from build123d import *

# Parameters (mm, degrees)
F1_DEPTH = 1
F3_W     = 140
F3_H     = 1
F4_DEPTH = 2
F6_DEPTH = 1


with BuildPart() as f1:
    # F0 (on Top) → F1 (new body)
    with BuildSketch(Plane.XY):
        Polygon((-20, 0), (0, 0), (0, 180), (-70, 180), (-70, 110), align=None)
        with BuildLine():
            ThreePointArc((-58.549692, 120), (-62.817459, 118.232233), (-61.049692, 122.5))
            ThreePointArc((-61.049692, 122.5), (-59.281925, 121.767767), (-58.549692, 120))
        make_face(mode=Mode.SUBTRACT)
        with BuildLine():
            ThreePointArc((-32.549692, 120), (-35.049692, 117.5), (-37.549692, 120))
            ThreePointArc((-37.549692, 120), (-36.817459, 121.767767), (-35.049692, 122.5))
            ThreePointArc((-35.049692, 122.5), (-33.281925, 121.767767), (-32.549692, 120))
        make_face(mode=Mode.SUBTRACT)
        with BuildLine():
            ThreePointArc((-61.049692, 170.5), (-62.817459, 174.767767), (-58.549692, 173))
            ThreePointArc((-58.549692, 173), (-59.281925, 171.232233), (-61.049692, 170.5))
        make_face(mode=Mode.SUBTRACT)
        with BuildLine():
            ThreePointArc((-32.549692, 173), (-33.281925, 171.232233), (-35.049692, 170.5))
            ThreePointArc((-35.049692, 170.5), (-36.817459, 174.767767), (-32.549692, 173))
        make_face(mode=Mode.SUBTRACT)
    extrude(amount=F1_DEPTH)

    # F2: F1 across face


with BuildPart() as f1_1:
    add(f1.part)
    add(f1.part.mirror(Plane(origin=(0, 90, 0.5), x_dir=(0, 1, 0), z_dir=(1, 0, 0))))

    # F3 (on face) → F4 (join)
    with BuildSketch(Plane.XY.offset(1)):
        with Locations((0, 179.5)):
            Rectangle(F3_W, F3_H)
    extrude(amount=F4_DEPTH)

    # F5 (on face) → F6 (join)
    with BuildSketch(Plane.XY.offset(1)):
        Polygon((-69, 110.216609), (-69, 179), (-70, 179), (-70, 110), (-20, 0), (-16.780434, 0), (16.780434, 0), (20, 0), (70, 110), (70, 179), (69, 179), (69, 110.216609), (19.356087, 1), (-19.356087, 1), align=None)
    extrude(amount=F6_DEPTH)


solid = f1_1.part
Read the model definition and answer for the solid it produces. Units are mm, in the model's axes. A direction names the side the tool comes from. Coordinates: 2 decimals unless noted, no trailing zeros. Order: outer loops, then holes, each group sorted by start corner. A loop starts at its lowest first (then second) coordinate and runs counter-clockwise, first axis right, second up. Notation, with made-up numbers: M 18,-23 L 59,-23 A17 ccw 59,-14 Z; hole C 57,6.5 d5. An arc over 180 degrees is marked long. Put each result on its own line as item: value. Start each with the question number.
Item 1: Section B-B, the plane x = 50 is taken. Determine the outline of the cut face in (y, z).
Item 2: Section A-A, the plane y = 88 is taken. Determine the outline of the cut face in (x, z), plus the area to 3 significant figures.
Item 3: Consider probe 1 along X at (y, z) = (173, 0.5); probe 2 along X at (y, z) = (171.5, 1.2); probe 3 along Y at (x, z) = (23.5, 2.85). Determine where each line is inside the solid, lowest interval first. Write a range as [from, to].
Item 4: Given pin 1 Ø3 at (x, y) = (35.05, 173) entering from -Z; pin 2 Ø1.5 at (x, z) = (-27.5, 1.5) entering from -Y; pin 3 Ø10 at (x, y) = (15.5, 118) entering from +Z, each flat-ended and moving along its own axis, determine where each tip first touches the part or whether it passes through.
Item 5: For faces 4 (the face through (44.526, 56.373, 1.493)), 5 (the face through (44.65, 54.23, 0.99)), determine the directions among +Z, -Z, +X, -X, +Y, -Y from which every point of the face is accessible in a straight line to the end or side of a thin tool.
Item 6: The mould has two halves that part along Y. Classify faces 1 (the face through (-45.35, 55.77, 0.99)), 2 (the face through (1, 111, 0)), 3 (the face through (-43.83, 54.84, 1.49)): +Y half, -Y half, draft (parallel to the pull), parting line (faces both ways), or undercut.
Computed:
1. outline: M 66,0 L 180,0 L 180,3 L 179,3 L 179,1 L 68.42,1 L 68.42,2 L 66,2 Z
2. outline: M -60,0 L 60,0 L 60,2 L 58.9,2 L 58.9,1 L -58.9,1 L -58.9,2 L -60,2 Z
2. area: 122 mm2
3. probe 1: x = [-70, -63.55], [-58.55, -37.55], [-32.55, 32.55], [37.55, 58.55], [63.55, 70]
3. probe 2: x = [-70, -69], [69, 70]
3. probe 3: y = [179, 180]
4. pin 1: passes through
4. pin 2: stops at y = 14.85
4. pin 3: stops at z = 1
5. face 4: +Z
5. face 5: +Z, -Z, +X, -Y
6. face 1: -Y half
6. face 2: draft
6. face 3: undercut
